Drawing for the job (mm, zero at the part's lowest x, y, z). Give positions to 0.01 mm unless a question says otherwise; leave off trailing zeros. Order: outer loops, then holes, each group sorted by start corner. A loop starts at its lowest first (then second) coordinate and runs counter-clockwise, first axis right, second up. Notation, with made-up numbers: (42, 56) - (88, 56) arc R19 ccw to (88, 62) - close; hole circle Ø6 at (-26, 31.5). An arc over 180 degrees is marked (long way). Use CSV: the item, a comma, the result in double quotes. Start each with the question number.
(1) Probe L1, parallel to X at y = 1, z = 12.7; L2, parallel to X at y = 0.35, z = 11.75 (1 decimal); L3, parallel to Z at x = 12.7, y = 0.55. List the from-to ranges inside material, lowest first.
(2) Drop flat-ended pins along their axis: pin 1 Ø4.5 at (x, z) = (38.1, 12.7) entering from +Y; pin 2 Ø1.2 at (x, z) = (22.86, 9.525) entering from +Y. Give the stop position or say it passes through.
(3) Band-saw the part on B-B, the plane z = 12.7. Give the cut face in (x, y).
(4) Band-saw the part on C-C, the plane x = 27.94. Give the cut face in (y, z) (1 decimal).
(5) Band-saw the part on A-A, the plane x = 38.1. Give the cut face in (y, z).
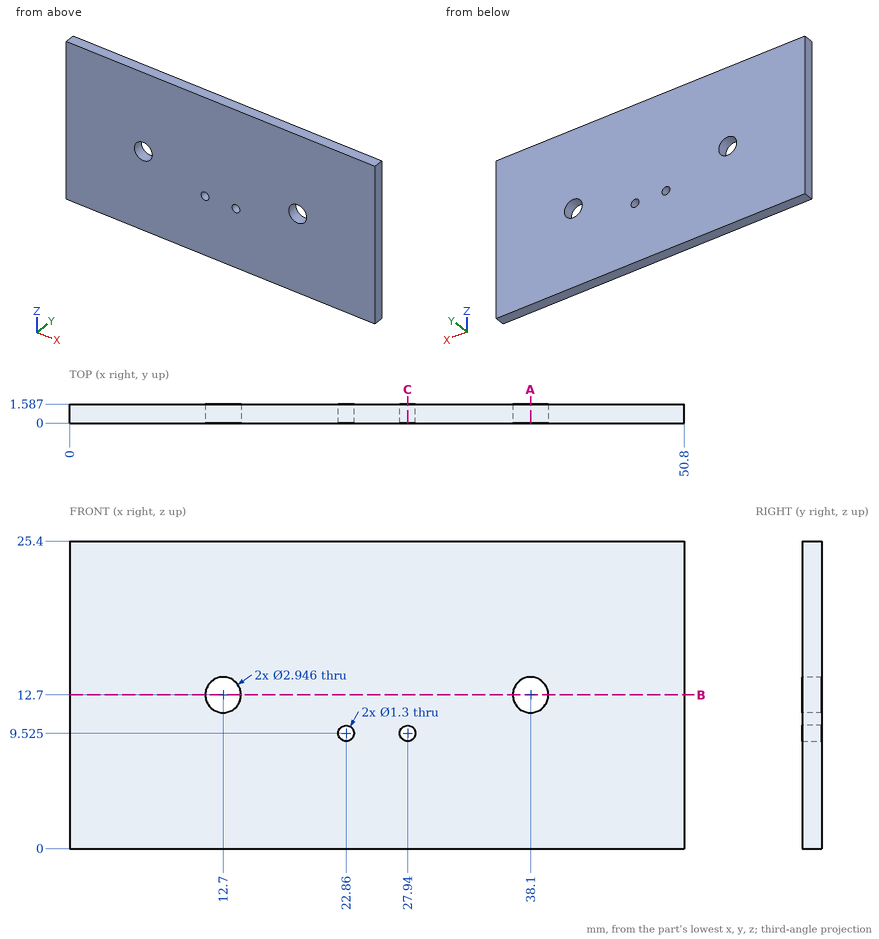
Answer block:
1,L1,"x = 0 to 11.23, 14.17 to 36.63, 39.57 to 50.8"
1,L2,"x = 0 to 11.6, 13.8 to 37, 39.2 to 50.8"
1,L3,"z = 0 to 11.23, 14.17 to 25.4"
2,pin 1,"stops at y = 1.59"
2,pin 2,"passes through"
3,outline,"(0, 0) - (11.23, 0) - (11.23, 1.59) - (0, 1.59) - close; (14.17, 0) - (36.63, 0) - (36.63, 1.59) - (14.17, 1.59) - close; (39.57, 0) - (50.8, 0) - (50.8, 1.59) - (39.57, 1.59) - close"
4,outline,"(0, 0) - (1.6, 0) - (1.6, 8.9) - (0, 8.9) - close; (0, 10.2) - (1.6, 10.2) - (1.6, 25.4) - (0, 25.4) - close"
5,outline,"(0, 0) - (1.59, 0) - (1.59, 11.23) - (0, 11.23) - close; (0, 14.17) - (1.59, 14.17) - (1.59, 25.4) - (0, 25.4) - close"
